from build123d import *

# Parameters (mm, degrees)
SKETCH1_R               = 92.71
SKETCH1_R_2             = 53.975
TOP_OF_HATCH_DEPTH      = 3.302
SKETCH2_R               = 92.71
SKETCH2_R_2             = 89.662
HATCH_BODY_DEPTH        = 259.08
SKETCH3_R               = 13.335
CHARGE_TUBE_HOLES_DEPTH = 263.382
SKETCH4_R               = 3.81
BOLT_HOLES_DEPTH        = 263.382
SKETCH_5_R              = 5.08
ANTENNA_HOLES_DEPTH     = 263.382


with BuildPart() as part:
    # Sketch1 → Top of Hatch (new body)
    with BuildSketch(Plane(origin=(0, 0, 0), x_dir=(1, 0, 0), z_dir=(0, 1, 0))):
        Circle(SKETCH1_R)
        Circle(SKETCH1_R_2, mode=Mode.SUBTRACT)
    extrude(amount=TOP_OF_HATCH_DEPTH)

    # Sketch2 → Hatch Body (add)
    with BuildSketch(Plane(origin=(0, 3.302, 0), x_dir=(1, 0, 0), z_dir=(0, 1, 0))):
        Circle(SKETCH2_R)
        Circle(SKETCH2_R_2, mode=Mode.SUBTRACT)
    extrude(amount=HATCH_BODY_DEPTH)

    # Sketch3 → Charge Tube Holes (cut, through all)
    with BuildSketch(Plane.XZ):
        with Locations((-76.454, 0)):
            Circle(SKETCH3_R)
        with Locations((76.454, 0)):
            Circle(SKETCH3_R)
    extrude(amount=-CHARGE_TUBE_HOLES_DEPTH, mode=Mode.SUBTRACT)

    # Sketch4 → Bolt Holes (cut, through all)
    with BuildSketch(Plane.XZ):
        with Locations((38.1, 65.991135768)):
            Circle(SKETCH4_R)
        with Locations((-38.1, 65.991135768)):
            Circle(SKETCH4_R)
        with Locations((-38.1, -65.991135768)):
            Circle(SKETCH4_R)
        with Locations((38.1, -65.991135768)):
            Circle(SKETCH4_R)
    extrude(amount=-BOLT_HOLES_DEPTH, mode=Mode.SUBTRACT)

    # Sketch 5 → Antenna Holes (cut, through all)
    with BuildSketch(Plane.XZ):
        with Locations((-26.112352144, 57.324838678)):
            Circle(SKETCH_5_R)
        with Locations((9.193647856, 61.033450854)):
            Circle(SKETCH_5_R)
    extrude(amount=-ANTENNA_HOLES_DEPTH, mode=Mode.SUBTRACT)


solid = part.part
Check sheet for the modelled part. Datum: model origin and axes. Units: mm. A direction names the side the tool comes from. Round coordinates to 2 decimals unless told otherwise and drop trailing zeros. Order: outer loops, then holes, each group sorted by start corner. A loop starts at its lowest first (then second) coordinate and runs counter-clockwise, first axis right, second up. Notation, with made-up numbers: M 24.25,-19 L 67.25,-19 A17 cw 67.25,0 Z; hole C 23.25,17 d8. An arc over 180 degrees is marked long. One line per item, written item: value. Start each with the question number.
1. Gauge pin test, flat ends, axial feed: P1, Ø3, axis at y = 155, z = 20, coming from the +X side; P2, Ø3, axis at y = 114.5, z = 64, coming from the +X side; P3, Ø12, axis at y = 91.5, z = 14.5, coming from the -X side. Record the tip position at first contact, or that the pin passes through.
2. Access from +Z, -Z, +X, -X, +Y, -Y to the whole of each face (thin tool, end or side, straight path). Record for faces 4 (the cylindrical face through (37.604, 1.628, -62.214)), 5 (the cylindrical face through (-1.94, 131.03, 89.64)).
3. Release check for a two-part mould opening along Z. For faces 1 (the flat face through (-35, 262.382, -83)), 2 (the cylindrical face through (85.64, 129.35, 35.51)), 3 (the cylindrical face through (35.292, 1.628, 68.566)) record: released by +Z, released by -Z, zero draft, split by the parting line, or undercut.
4. Section check B-B on z = 31.5. Enter the section's corners in (x, y), and give its area (3 significant figures).
5. Section check C-C on y = 118.5. Enter the section's corners in (x, z) (3 decimals).
6. Section check D-D on x = -38.1. Enter the section's corners in (y, z).
7. Section check A-A on x = 0. Enter the section's corners in (y, z) (3 decimals).
8. Scan lines: line 1 along X through (y, z) = (186, 0); line 2 along Y through (x, z) = (-24, -73.5); line 3 along Z through (x, y) = (-19, 14.5). Record each from-to range of solid material in increasing order.
Results found:
1. P1: x = 90.85
1. P2: x = 68.48
1. P3: x = -92.32
2. face 4: +Y, -Y
2. face 5: +Y
3. face 1: zero draft
3. face 2: split by the parting line
3. face 3: undercut
4. outline: M -87.19,0 L -43.83,0 L -43.83,3.3 L -83.95,3.3 L -83.95,262.38 L -87.19,262.38 Z; M 43.83,0 L 87.19,0 L 87.19,262.38 L 83.95,262.38 L 83.95,3.3 L 43.83,3.3 Z
4. area: 1,970 mm^2
5. outline: C 0,0 d185.42; hole M -89.64,-1.988 A89.662 ccw 89.64,-1.988 A13.335 ccw 89.64,1.988 A89.662 ccw -89.64,1.988 A13.335 ccw Z
6. outline: M 0,-84.52 L 262.38,-84.52 L 262.38,-81.16 L 3.3,-81.16 L 3.3,-69.8 L 0,-69.8 Z; M 0,-62.18 L 3.3,-62.18 L 3.3,-38.23 L 0,-38.23 Z; M 0,38.23 L 3.3,38.23 L 3.3,62.18 L 0,62.18 Z; M 0,69.8 L 3.3,69.8 L 3.3,81.16 L 262.38,81.16 L 262.38,84.52 L 0,84.52 Z
7. outline: M 0,-92.71 L 262.382,-92.71 L 262.382,-89.662 L 3.302,-89.662 L 3.302,-53.975 L 0,-53.975 Z; M 0,53.975 L 3.302,53.975 L 3.302,89.662 L 262.382,89.662 L 262.382,92.71 L 0,92.71 Z
8. line 1: -92.71 to -89.79, 89.79 to 92.71
8. line 2: 0 to 3.3
8. line 3: -90.74 to -87.63, 87.63 to 90.74
